Could you check a few things on this model? Use its own coordinates, in mm. A direction names the side the tool comes from. Coordinates: 2 decimals unless noted, no trailing zeros. Write each loop counter-clockwise with the first axis right and the second up, starting at its lowest first coordinate (ties: lowest second). Pieces come first, ordered by that corner, then holes.
Item 1: I want a section at A-A on x = -29.5. Please give me the cut outline in (y, z).
Item 2: I want a section at D-D on x = 7.5. Please give me the cut outline in (y, z), then the cut area to 3 significant figures.
Item 3: If I drill on probe 1 along Y at (x, z) = (-16.5, 3); probe 2 along Y at (x, z) = (-30, -3.5); probe 3 along Z at (x, y) = (-11.5, 54.5), over which ranges is the centre line in solid material (lowest first)?
Item 4: Thinking about a two-plate mould opening in Y: for faces 4 (the flat face through (9.9, 25, -10)), 5 (the flat face through (-17, 58.8, 15)), 6 (the flat face through (-39.5, 5, 0.2)), which applies, +Y half, -Y half, draft (parallel to the pull), parting line (faces both ways), or undercut?
Item 5: Which directions (+Z, -Z, +X, -X, +Y, -Y) give clear straight access to the entire face, cutting with the end or side of a thin tool? Please do faces 1 (the flat face through (9.9, 13, -2)), 2 (the flat face through (-14, 35.8, -4)), 3 (the flat face through (-14, 47, 4)).
Item 6: For P1, Ø2, axis at x = -7, y = 6, coming from the -Z side; P2, Ø8, axis at x = -9, y = 7.5, coming from the +Z side; P3, Ø1.2, axis at y = 21.5, z = -9.5, coming from the -X side, each with a flat end and sliding along its axis, tell me the tip position at first contact or that it passes through.
Item 7: I want a section at B-B on z = -7. Please give me the cut outline in (x, y), then the cut area to 3 significant figures.
Item 8: I want a section at C-C on y = 42. Please give me the cut outline in (x, z).
from build123d import *

# Parameters (mm, degrees)
SKETCH_1_W       = 11.8
SKETCH_1_H       = 22.8
EXTRUDE_1_DEPTH  = 4
SKETCH_2_W       = 15.8
SKETCH_2_H       = 4
EXTRUDE_2_DEPTH  = 2
SKETCH_5_W       = 15.8
SKETCH_5_H       = 4
EXTRUDE_4_DEPTH  = 2
SKETCH_6_W       = 15.8
SKETCH_6_H       = 4
EXTRUDE_5_DEPTH  = 11.8
SKETCH_7_W       = 4
SKETCH_7_H       = 14.2
EXTRUDE_7_DEPTH  = 4
SKETCH_8_W       = 4
SKETCH_8_H       = 22.8
EXTRUDE_8_DEPTH  = 33.6
SKETCH_10_W      = 15.8
SKETCH_10_H      = 4
EXTRUDE_9_DEPTH  = 33.6
SKETCH_11_W      = 15.8
SKETCH_11_H      = 4
EXTRUDE_10_DEPTH = 33.6
SKETCH_12_W      = 45.4
SKETCH_12_H      = 3.8
EXTRUDE_11_DEPTH = 22.8


with BuildPart() as part:
    # 스케치1 → 보스-돌출1 (new body)
    with BuildSketch(Plane.XY):
        Rectangle(SKETCH_1_W, SKETCH_1_H)
    extrude(amount=EXTRUDE_1_DEPTH)

    # 스케치2 → 보스-돌출2 (add)
    with BuildSketch(Plane(origin=(0, 11.4, 0), x_dir=(1, 0, 0), z_dir=(0, 1, 0))):
        with Locations((2, -2)):
            Rectangle(SKETCH_2_W, SKETCH_2_H)
    extrude(amount=EXTRUDE_2_DEPTH)

    # 스케치5 → 보스-돌출4 (add)
    with BuildSketch(Plane(origin=(0, 13.4, 0), x_dir=(1, 0, 0), z_dir=(0, 1, 0))):
        with Locations((2, -2)):
            Rectangle(SKETCH_5_W, SKETCH_5_H)
    extrude(amount=EXTRUDE_4_DEPTH)

    # 스케치6 → 보스-돌출5 (add)
    with BuildSketch(Plane(origin=(0, 0, 0), x_dir=(-1, 0, 0), z_dir=(0, 0, -1))):
        with Locations((-2, 13.4)):
            Rectangle(SKETCH_6_W, SKETCH_6_H)
    extrude(amount=EXTRUDE_5_DEPTH)

    # 스케치7 → 보스-돌출7 (add)
    with BuildSketch(Plane(origin=(9.9, 0, 0), x_dir=(0, 0, -1), z_dir=(1, 0, 0))):
        with Locations((9.8, 18.5)):
            Rectangle(SKETCH_7_W, SKETCH_7_H)
    extrude(amount=EXTRUDE_7_DEPTH)

    # 스케치8 → 보스-돌출8 (add)
    with BuildSketch(Plane.ZY.offset(5.9)):
        with Locations((2, 0)):
            Rectangle(SKETCH_8_W, SKETCH_8_H)
    extrude(amount=EXTRUDE_8_DEPTH)

    # 대칭 복사3: part across plane


with BuildPart() as part_1:
    add(part.part)
    add(part.part.mirror(Plane(origin=(13.9, 25.6, -11.8), x_dir=(0, 0, 1), z_dir=(0, -1, 0))))

    # 스케치10 → 보스-돌출9 (add)
    with BuildSketch(Plane.ZY.offset(5.9)):
        with Locations((-3.9, 13.4)):
            Rectangle(SKETCH_10_W, SKETCH_10_H)
    extrude(amount=EXTRUDE_9_DEPTH)

    # 스케치11 → 보스-돌출10 (add)
    with BuildSketch(Plane.ZY.offset(5.9)):
        with Locations((-3.9, 37.8)):
            Rectangle(SKETCH_11_W, SKETCH_11_H)
    extrude(amount=EXTRUDE_10_DEPTH)

    # 스케치12 → 보스-돌출11 (add)
    with BuildSketch(Plane.XY.offset(4)):
        with Locations((-16.8, 60.7)):
            Rectangle(SKETCH_12_W, SKETCH_12_H)
    extrude(amount=EXTRUDE_11_DEPTH)


solid = part_1.part
Response values:
1. outline: (-11.4, 0) - (11.4, 0) - (11.4, -11.8) - (15.4, -11.8) - (15.4, 4) - (-11.4, 4) - close; (35.8, -11.8) - (39.8, -11.8) - (39.8, 0) - (62.6, 0) - (62.6, 26.8) - (58.8, 26.8) - (58.8, 4) - (35.8, 4) - close
2. outline: (11.4, -11.8) - (15.4, -11.8) - (15.4, 4) - (11.4, 4) - close; (35.8, -11.8) - (39.8, -11.8) - (39.8, 4) - (35.8, 4) - close
2. area: 126 mm2
3. probe 1: y = -11.4 to 15.4, 35.8 to 62.6
3. probe 2: y = 11.4 to 15.4, 35.8 to 39.8
3. probe 3: z = 0 to 4
4. face 4: undercut
4. face 5: -Y half
4. face 6: draft
5. face 1: +Z, +X, +Y, -Y
5. face 2: +Z, -Z, -X
5. face 3: +Z, +X, -X, -Y
6. P1: stops at z = 0
6. P2: stops at z = 4
6. P3: stops at x = 9.9
7. outline: (-39.5, 11.4) - (9.9, 11.4) - (9.9, 15.4) - (-39.5, 15.4) - close; (-39.5, 35.8) - (9.9, 35.8) - (9.9, 39.8) - (-39.5, 39.8) - close
7. area: 395 mm2
8. outline: (-39.5, 0) - (5.9, 0) - (5.9, 4) - (-39.5, 4) - close
